Design review of the part shown in the three views and the two pictorial views. Dimensions are in mm from the part's minimum x, y and z. Coordinates: 2 decimals unless noted, no trailing zeros. Loops run counter-clockwise (first coordinate to the right, second up) from the corner with the lowest first, then second, coordinate; pieces in that order, holes last.
Q1. Add section C-C on y = 1.95. Give the boundary of the cut face in (x, z).
Q2. Add section B-B on x = 4. Give the boundary of the cut face in (y, z).
Q3. Wall thickness on probe 1 along Z at (x, y) = (36, 3.65); probe 2 along X at (y, z) = (2.1, 71); probe 3 along Z at (x, y) = (20, 2.1): over which ranges is each line inside the solid? List them lowest first.
Q4. Add section A-A on z = 71. Give the boundary of the cut face in (x, y).
Q5. Add section D-D on x = 20. Give the boundary of the cut face in (y, z), and give its area (3 significant figures).
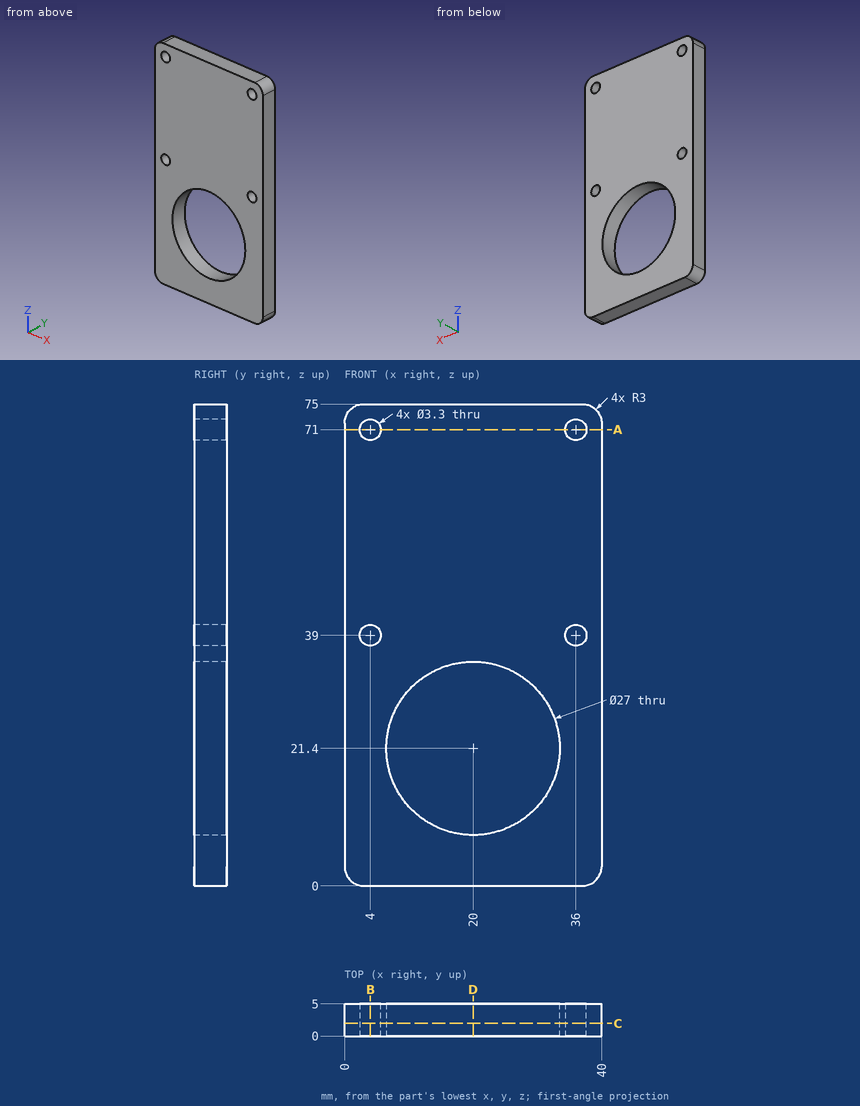
Entries:
1. outline: (0, 3) arc R3 ccw to (3, 0) - (37, 0) arc R3 ccw to (40, 3) - (40, 72) arc R3 ccw to (37, 75) - (3, 75) arc R3 ccw to (0, 72) - close; hole circle Ø3.3 at (4, 39); hole circle Ø3.3 at (4, 71); hole circle Ø27 at (20, 21.4); hole circle Ø3.3 at (36, 39); hole circle Ø3.3 at (36, 71)
2. outline: (0, 0) - (5, 0) - (5, 37.35) - (0, 37.35) - close; (0, 40.65) - (5, 40.65) - (5, 69.35) - (0, 69.35) - close; (0, 72.65) - (5, 72.65) - (5, 75) - (0, 75) - close
3. probe 1: z = 0 to 37.35, 40.65 to 69.35, 72.65 to 75
3. probe 2: x = 0 to 2.35, 5.65 to 34.35, 37.65 to 40
3. probe 3: z = 0 to 7.9, 34.9 to 75
4. outline: (0, 0) - (2.35, 0) - (2.35, 5) - (0, 5) - close; (5.65, 0) - (34.35, 0) - (34.35, 5) - (5.65, 5) - close; (37.65, 0) - (40, 0) - (40, 5) - (37.65, 5) - close
5. outline: (0, 0) - (5, 0) - (5, 7.9) - (0, 7.9) - close; (0, 34.9) - (5, 34.9) - (5, 75) - (0, 75) - close
5. area: 240 mm2
